Can you work these out from the model? Positions are in its coordinate system, mm. Face numbers are marked on the shaded views. Round coordinates to 2 decimals unless told otherwise and drop trailing zeros. Loops run counter-clockwise (first coordinate to the right, second up) from the corner with the lowest first, then second, coordinate; pieces in that order, holes last. Notation, with made-up numbers: (66, 14) -> (98, 14) arc R35 ccw to (98, 51) -> close; hole circle Ø9 at (69, -18). An arc over 180 degrees is marked (long way). Answer as a JSON object with one key per item and string values.
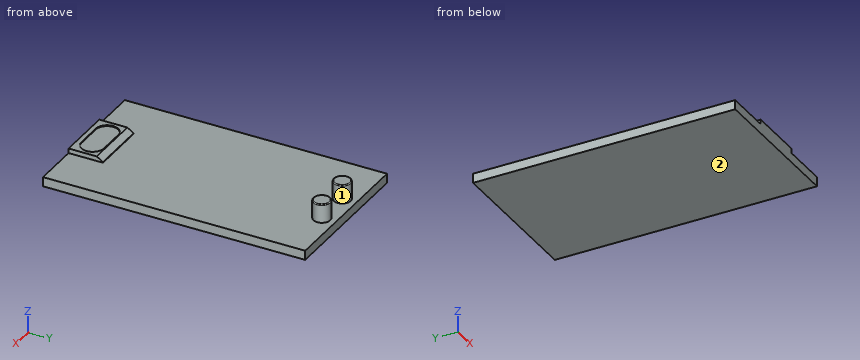
```python
from build123d import *

# Parameters (mm, degrees)
F0_W     = 203.2
F0_H     = 355.6
F1_DEPTH = 12.7
F2_R     = 11.43
F3_DEPTH = 38.1
F4_W     = 76.2
F4_H     = 38.1
F5_DEPTH = 6.35
F7_DEPTH = 1.27
F9_DEPTH = 76.2
F10_R    = 1.27


with BuildPart() as f1:
    # F0 (on Top) → F1 (new body)
    with BuildSketch(Plane.XY):
        with Locations((101.6, 177.8)):
            Rectangle(F0_W, F0_H)
    extrude(amount=F1_DEPTH)

    # F2 (on face) → F3 (join)
    with BuildSketch(Plane.XY):
        with Locations((76.2, 336.55)):
            Circle(F2_R)
        with Locations((127, 336.55)):
            Circle(F2_R)
    extrude(amount=F3_DEPTH)

    # F4 (on face) → F5 (join)
    with BuildSketch(Plane.XY.offset(12.7)):
        with Locations((101.6, 19.05)):
            Rectangle(F4_W, F4_H)
    extrude(amount=F5_DEPTH)

    # F6 (on face) → F7 (cut)
    with BuildSketch(Plane.XY.offset(19.05)):
        with BuildLine():
            Line((119.38, 36.83), (83.82, 36.83))
            ThreePointArc((83.82, 36.83), (68.58, 21.59), (83.82, 6.35))
            Line((83.82, 6.35), (119.38, 6.35))
            ThreePointArc((119.38, 6.35), (134.62, 21.59), (119.38, 36.83))
        make_face()
    extrude(amount=-F7_DEPTH, mode=Mode.SUBTRACT)

    # F8 (on face) → F9 (join)
    with BuildSketch(Plane.YZ.offset(139.7)):
        Polygon((46.687422, 13.682861), (38.1, 19.05), (38.1, 12.7), (46.687422, 12.7), align=None)
    extrude(amount=-F9_DEPTH)

    # F10
    f10_edges = [f1.edges().sort_by_distance(p)[0] for p in [
        (64.77, 336.55, 38.1),
        (115.57, 336.55, 38.1),
    ]]
    fillet(f10_edges, radius=F10_R)


solid = f1.part
```
Q1. If I drill on L1, parallel to Z at x = 19.5, y = 75; L2, parallel to Y at x = 127.5, z = 36.5; L3, parallel to Y at x = 88.5, z = 18, over which ranges is the centre line in solid material (lowest first)? Write a range as [from, to].
Determined:
{"L1": "[0, 12.7]", "L2": "[325.13, 347.97]", "L3": "[0, 6.35], [36.83, 39.78]"}
Q2. I want a section at A-A, the plane y = 21.59. Write out the boundary of the cut face in (x, z).
Determined:
{"outline": "(0, 0) -> (203.2, 0) -> (203.2, 12.7) -> (139.7, 12.7) -> (139.7, 19.05) -> (134.62, 19.05) -> (134.62, 17.78) -> (68.58, 17.78) -> (68.58, 19.05) -> (63.5, 19.05) -> (63.5, 12.7) -> (0, 12.7) -> close"}
Q3. I'm going to push flat-ended pins straight in: pin 1 (3 mm diameter, centred on y = 21, z = 17, fed in from -X); pin 2 (0.8 mm diameter, centred on x = 111.5, z = 13, fed in from +Y); pin 3 (5 mm diameter, centred on x = 104, z = 22.5, fed in from +Y); pin 4 (2 mm diameter, centred on x = 121.5, y = 169, fed in from +Z). Where does each tip first touch, or does it pass through?
Determined:
{"pin 1": "x = 63.5", "pin 2": "y = 355.6", "pin 3": "through", "pin 4": "z = 12.7"}
Q4. I want a section at C-C, the plane x = 127. Write out the boundary of the cut face in (y, z).
Determined:
{"outline": "(0, 0) -> (355.6, 0) -> (355.6, 12.7) -> (347.98, 12.7) -> (347.98, 36.83) arc R1.27 ccw to (346.71, 38.1) -> (326.39, 38.1) arc R1.27 ccw to (325.12, 36.83) -> (325.12, 12.7) -> (46.69, 12.7) -> (46.69, 13.68) -> (38.1, 19.05) -> (34.79, 19.05) -> (34.79, 17.78) -> (8.39, 17.78) -> (8.39, 19.05) -> (0, 19.05) -> close"}
Q5. We'd pull the mould along X, two halves only. Please class the marked faces 1 and 2: pulls with the +X half, pulls with the -X half, needs draft (parallel to the pull), parting line crosses it, or undercut.
Determined:
{"face 1": "undercut", "face 2": "needs draft"}
Q6. I want a section at D-D, the plane y = 336.55. Write out the boundary of the cut face in (x, z).
Determined:
{"outline": "(0, 0) -> (203.2, 0) -> (203.2, 12.7) -> (138.43, 12.7) -> (138.43, 36.83) arc R1.27 ccw to (137.16, 38.1) -> (116.84, 38.1) arc R1.27 ccw to (115.57, 36.83) -> (115.57, 12.7) -> (87.63, 12.7) -> (87.63, 36.83) arc R1.27 ccw to (86.36, 38.1) -> (66.04, 38.1) arc R1.27 ccw to (64.77, 36.83) -> (64.77, 12.7) -> (0, 12.7) -> close"}
Q7. I want a section at B-B, the plane z = 27. Write out the boundary of the cut face in (x, y), then the cut area to 3 significant figures.
Determined:
{"outline": "circle Ø22.86 at (76.2, 336.55); circle Ø22.86 at (127, 336.55)", "area": "821 mm²"}
